Geometry check sheet. Reference: drawing and pictorial views, mm from the part's lowest x, y, z. Give positions to 0.01 mm unless a question says otherwise; leave off trailing zeros. Write each loop counter-clockwise with the first axis right and the second up, starting at its lowest first coordinate (ties: lowest second). Pieces come first, ordered by that corner, then holes. Notation, with made-up numbers: M 33.5,-30 L 58.5,-30 A22 ccw 58.5,-14 Z; hole C 70,36.25 d2. An arc over 180 degrees is marked long. One line per item, written item: value. Start each with the question number.
1. Gauge pin test, flat ends, axial feed: pin 1 (1 mm diameter, centred on y = 107, z = 1.5, fed in from +X); pin 2 (1.5 mm diameter, centred on y = 59, z = 1, fed in from +X) (1 decimal). Record the tip position at first contact, or that the pin passes through.
2. Scan lines: line 1 (Y direction, x = 179.5, z = 1.3); line 2 (Y direction, x = 186, z = 1.9) (1 decimal); line 3 (X direction, y = 90, z = 1.05). Record each from-to range of solid material in increasing order.
3. Cross-section at B-B on y = 80.5. Record the cut outline in (x, z) (1 decimal).
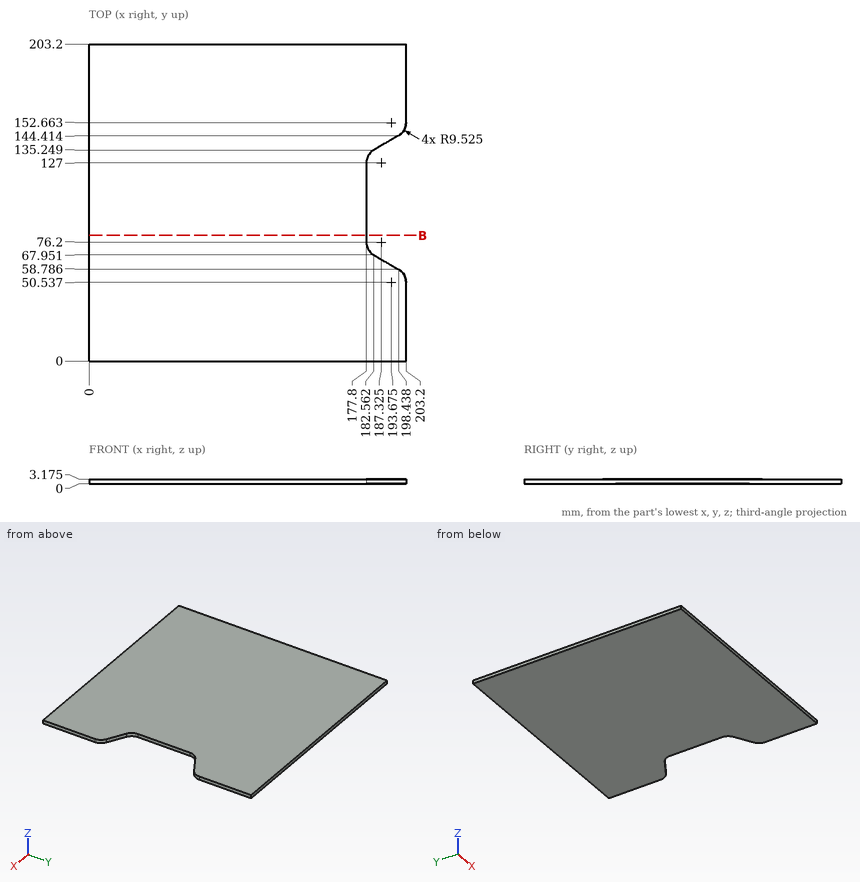
Report:
1. pin 1: stops at x = 177.8
1. pin 2: stops at x = 199.3
2. line 1: y = 0 to 70.77, 132.43 to 203.2
2. line 2: y = 0 to 66, 137.2 to 203.2
2. line 3: x = 0 to 177.8
3. outline: M 0,0 L 177.8,0 L 177.8,3.2 L 0,3.2 Z
